Work out the finished part from the listing and answer in its coordinate system (mm). A direction names the side the tool comes from. Round coordinates to 2 decimals unless told otherwise and drop trailing zeros. Loops run counter-clockwise (first coordinate to the right, second up) from the corner with the lowest first, then second, coordinate; pieces in that order, holes last. Notation, with made-up numbers: (62, 72) - (97, 72) arc R25 ccw to (97, 103) - close; hole circle Ø11 at (79, 86). An arc over 180 degrees is marked (long way). Answer as CSV lines item,"result". Start each with the question number.
Q1. Section C-C on z = 32 is taken. Write down the section's boundary in (x, y), then the cut area to 3 significant figures.
Q2. Section A-A on x = 69.5 is taken. Write down the section's boundary in (y, z).
Q3. The mould has two halves that part along Y. Classify faces 3 (the face through (-112.39, 4.95, 9.86)), 4 (the face through (-97.5, -0.5, 9.9)): +Y half, -Y half, draft (parallel to the pull), parting line (faces both ways), or undercut.
Q4. Section D-D on z = 69 is taken. Write down the section's boundary in (x, y).
Q5. For faces 1 (the face through (-33.766, 25.891, 4.93)), 2 (the face through (46.5, -0.65, 9.86)), determine the directions among +Z, -Z, +X, -X, +Y, -Y from which every point of the face is accessible in a straight line to the end or side of a thin tool.
Q6. Section B-B on y = -62.5 is taken. Write down the section's boundary in (x, z).
Q7. Straight lines are drawn through the part: L1, parallel to Y at x = 0, z = 4.25; L2, parallel to Y at x = 0, z = 39; L3, parallel to Y at x = -71, z = 5.5. For each, find the intervals that lie inside material, in ascending order. Write a range as [from, to].
Q8. Each of these flat-tipped pins is pushed along its axis until it touches: pin 1 Ø6 at (y, z) = (78, 12) entering from +X; pin 2 Ø16 at (y, z) = (-63.5, 13.5) entering from -X; pin 3 Ø10 at (x, y) = (27.5, -4) entering from -Z. Where does it stop, or does it pass through?
```python
from build123d import *

# Parameters (mm, degrees)
F0_R     = 112.5
F1_DEPTH = 20
F4_R     = 19.05
F5_DEPTH = 90
F6_R     = 42.55
F7_DEPTH = 10


with BuildPart() as f1:
    # F0 (on Top) → F1 (new body)
    with BuildSketch(Plane.XY):
        Circle(F0_R)
        with BuildLine():
            ThreePointArc((-47.443954, -77.196073), (-57.151446, -78.373088), (-58.563792, -68.697033))
            Line((-58.563792, -68.697033), (-36.815737, -38.763404))
            ThreePointArc((-36.815737, -38.763404), (-27.037496, -37.215236), (-25.490409, -46.993649))
            Line((-25.490409, -46.993649), (-47.046201, -76.648867))
            ThreePointArc((-47.046201, -76.648867), (-47.238463, -76.927278), (-47.443954, -77.196073))
        make_face(mode=Mode.SUBTRACT)
        with BuildLine():
            ThreePointArc((-74.74068, -51.224927), (-84.08765, -48.351791), (-81.442286, -38.937822))
            Line((-81.442286, -38.937822), (-49.399346, -20.437822))
            ThreePointArc((-49.399346, -20.437822), (-39.836782, -23.00067), (-42.400686, -32.562951))
            Line((-42.400686, -32.562951), (-74.154746, -50.886811))
            ThreePointArc((-74.154746, -50.886811), (-74.443626, -51.062951), (-74.74068, -51.224927))
        make_face(mode=Mode.SUBTRACT)
        with BuildLine():
            ThreePointArc((-90.839791, -7.491748), (-97.497937, -0.330054), (-90.5, 6.5))
            Line((-90.5, 6.5), (-53.5, 6.5))
            ThreePointArc((-53.5, 6.5), (-46.5, -0.500773), (-53.501547, -7.5))
            Line((-53.501547, -7.5), (-90.163299, -7.491898))
            ThreePointArc((-90.163299, -7.491898), (-90.501547, -7.5), (-90.839791, -7.491748))
        make_face(mode=Mode.SUBTRACT)
        with BuildLine():
            ThreePointArc((6.991748, -91.339791), (-0.169946, -97.997937), (-7, -91))
            Line((-7, -91), (-7, -54))
            ThreePointArc((-7, -54), (0.000773, -47), (7, -54.001547))
            Line((7, -54.001547), (6.991898, -90.663299))
            ThreePointArc((6.991898, -90.663299), (7, -91.001547), (6.991748, -91.339791))
        make_face(mode=Mode.SUBTRACT)
        with BuildLine():
            ThreePointArc((58.75684, -68.97678), (56.876468, -78.572871), (47.237554, -76.926026))
            Line((47.237554, -76.926026), (25.489499, -46.992397))
            ThreePointArc((25.489499, -46.992397), (27.038747, -37.214327), (36.816646, -38.764656))
            Line((36.816646, -38.764656), (58.359329, -68.429399))
            ThreePointArc((58.359329, -68.429399), (58.564701, -68.698284), (58.75684, -68.97678))
        make_face(mode=Mode.SUBTRACT)
        with BuildLine():
            ThreePointArc((81.732428, -39.114864), (83.917705, -48.646146), (74.442286, -51.062178))
            Line((74.442286, -51.062178), (42.399346, -32.562178))
            ThreePointArc((42.399346, -32.562178), (39.837555, -22.99933), (49.400686, -20.438596))
            Line((49.400686, -20.438596), (81.146644, -38.776489))
            ThreePointArc((81.146644, -38.776489), (81.443626, -38.938596), (81.732428, -39.114864))
        make_face(mode=Mode.SUBTRACT)
        with BuildLine():
            ThreePointArc((90.839791, 6.491748), (97.497937, -0.669946), (90.5, -7.5))
            Line((90.5, -7.5), (53.5, -7.5))
            ThreePointArc((53.5, -7.5), (46.5, -0.499227), (53.501547, 6.5))
            Line((53.501547, 6.5), (90.163299, 6.491898))
            ThreePointArc((90.163299, 6.491898), (90.501547, 6.5), (90.839791, 6.491748))
        make_face(mode=Mode.SUBTRACT)
        with BuildLine():
            ThreePointArc((-88.078816, 21.266983), (-92.198004, 30.135639), (-83.431968, 34.468925))
            Line((-83.431968, 34.468925), (-48.242876, 23.035296))
            ThreePointArc((-48.242876, 23.035296), (-43.748839, 14.214046), (-52.570586, 9.720983))
            Line((-52.570586, 9.720983), (-87.43548, 21.057793))
            ThreePointArc((-87.43548, 21.057793), (-87.759677, 21.154612), (-88.078816, 21.266983))
        make_face(mode=Mode.SUBTRACT)
        with BuildLine():
            ThreePointArc((83.757678, 34.566078), (92.303036, 29.812383), (87.758205, 21.154134))
            Line((87.758205, 21.154134), (52.569114, 9.720505))
            ThreePointArc((52.569114, 9.720505), (43.748361, 14.215517), (48.244348, 23.035774))
            Line((48.244348, 23.035774), (83.11425, 34.357173))
            ThreePointArc((83.11425, 34.357173), (83.433439, 34.469403), (83.757678, 34.566078))
        make_face(mode=Mode.SUBTRACT)
        with BuildLine():
            ThreePointArc((7, 53), (-0.000773, 46), (-7, 53.001547))
            Line((-7, 53.001547), (-6.991898, 89.663299))
            ThreePointArc((-6.991898, 89.663299), (-7, 90.001547), (-6.991748, 90.339791))
            ThreePointArc((-6.991748, 90.339791), (0.169946, 96.997937), (7, 90))
            Line((7, 90), (7, 53))
        make_face(mode=Mode.SUBTRACT)
    extrude(amount=F1_DEPTH)

    # F2 (on Front) → F3 (revolve)
    with BuildSketch(Plane.XZ):
        Polygon((-40, 50), (-40, 20), (0, 20), (0, 90), (-25.441191, 90), align=None)
    revolve(axis=Axis((0, 0, 55), (0, 0, 1)))

    # F4 (on face) → F5 (cut, through all)
    with BuildSketch(Plane.XY.offset(90)):
        Circle(F4_R)
    extrude(amount=-F5_DEPTH, mode=Mode.SUBTRACT)

    # F6 (on face) → F7 (cut)
    with BuildSketch(Plane(origin=(0, 0, 0), x_dir=(1, 0, 0), z_dir=(0, 0, -1))):
        Circle(F6_R)
    extrude(amount=-F7_DEPTH, mode=Mode.SUBTRACT)


solid = f1.part
```
Findings:
1,outline,"circle Ø80 at (0, 0); hole circle Ø38.1 at (0, 0)"
1,area,"3,890 mm^2"
2,outline,"(-88.46, 0) - (-48.21, 0) - (-48.21, 20) - (-88.46, 20) - close; (-32.05, 0) - (-7.5, 0) - (-7.5, 20) - (-32.05, 20) - close; (6.5, 0) - (15.22, 0) - (15.22, 20) - (6.5, 20) - close; (29.94, 0) - (88.46, 0) - (88.46, 20) - (29.94, 20) - close"
3,face 3,"parting line"
3,face 4,"undercut"
4,outline,"circle Ø66.17 at (0, 0); hole circle Ø38.1 at (0, 0)"
5,face 1,"-Z"
5,face 2,"+Z, -Z"
6,outline,"(-93.54, 0) - (-54.06, 0) - (-54.06, 20) - (-93.54, 20) - close; (-36.76, 0) - (-7, 0) - (-7, 20) - (-36.76, 20) - close; (7, 0) - (36.76, 0) - (36.76, 20) - (7, 20) - close; (54.05, 0) - (93.54, 0) - (93.54, 20) - (54.05, 20) - close"
7,L1,"y = [-112.5, -98], [-47, -42.55], [42.55, 46], [97, 112.5]"
7,L2,"y = [-40, -19.05], [19.05, 40]"
7,L3,"y = [-87.27, -49.07], [-32.91, -7.5], [6.5, 15.71], [30.43, 87.27]"
8,pin 1,"stops at x = 83.85"
8,pin 2,"stops at x = -97.86"
8,pin 3,"stops at z = 10"
